from build123d import *

# Parameters (mm, degrees)
SKETCH1_R           = 7.95
BOSS_EXTRUDE1_DEPTH = 19.5
BOSS_EXTRUDE2_DEPTH = 1.5
SKETCH3_R           = 8.5
BOSS_EXTRUDE3_DEPTH = 2
BOSS_EXTRUDE3_TAPER = 30
SKETCH4_R           = 6
CUT_EXTRUDE1_DEPTH  = 2
SKETCH6_R           = 6
BOSS_EXTRUDE4_DEPTH = 2
BOSS_EXTRUDE4_TAPER = 30
SKETCH7_R           = 6.25
BOSS_EXTRUDE5_DEPTH = 9.3
SKETCH8_W           = 2.45599171
SKETCH8_H           = 0.676111723
SKETCH8_W_2         = 0.61301599
SKETCH8_H_2         = 2.333871056
SKETCH8_H_3         = 0.814342288
SKETCH8_W_3         = 0.602821575
BOSS_EXTRUDE6_DEPTH = 6


with BuildPart() as part:
    # Sketch1 → Boss-Extrude1 (new body)
    with BuildSketch(Plane(origin=(0, 0, 0), x_dir=(1, 0, 0), z_dir=(0, 1, 0))):
        with Locations(Location((0, 0, 0), (0, 0, 270))):
            Circle(SKETCH1_R)
    extrude(amount=BOSS_EXTRUDE1_DEPTH)

    # Sketch2 → Boss-Extrude2 (add)
    with BuildSketch(Plane(origin=(0, 19.5, 0), x_dir=(1, 0, 0), z_dir=(0, 1, 0))):
        Polygon((11.547005384, 0), (5.773502692, 10), (-5.773502692, 10), (-11.547005384, 0), (-5.773502692, -10), (5.773502692, -10), align=None)
    extrude(amount=-BOSS_EXTRUDE2_DEPTH)

    # Sketch3 → Boss-Extrude3 (add)
    with BuildSketch(Plane(origin=(0, 19.5, 0), x_dir=(1, 0, 0), z_dir=(0, 1, 0))):
        Circle(SKETCH3_R)
    extrude(amount=BOSS_EXTRUDE3_DEPTH, taper=BOSS_EXTRUDE3_TAPER)

    # Sketch4 → Cut-Extrude1 (cut)
    with BuildSketch(Plane(origin=(0, 21.5, 0), x_dir=(1, 0, 0), z_dir=(0, 1, 0))):
        with Locations(Location((0, 0, 0), (0, 0, 270))):
            Circle(SKETCH4_R)
    extrude(amount=-CUT_EXTRUDE1_DEPTH, mode=Mode.SUBTRACT)

    # Sketch6 → Boss-Extrude4 (add)
    with BuildSketch(Plane(origin=(0, 19.5, 0), x_dir=(1, 0, 0), z_dir=(0, 1, 0))):
        with Locations(Location((0, 0, 0), (0, 0, 270))):
            Circle(SKETCH6_R)
    extrude(amount=BOSS_EXTRUDE4_DEPTH, taper=BOSS_EXTRUDE4_TAPER)

    # Sketch7 → Boss-Extrude5 (add)
    with BuildSketch(Plane.XZ):
        with Locations(Location((0, 0, 0), (0, 0, 90))):
            Circle(SKETCH7_R)
    extrude(amount=BOSS_EXTRUDE5_DEPTH)

    # Sketch8 → Boss-Extrude6 (add)
    with BuildSketch(Plane.XZ.offset(9.3)):
        with Locations((0, 4.683948284)):
            Rectangle(SKETCH8_W, SKETCH8_H)
        with Locations((5.389572467, 0)):
            Rectangle(SKETCH8_W_2, SKETCH8_H_2)
        with Locations((0, -4.982726266)):
            Rectangle(SKETCH8_W, SKETCH8_H_3)
        with Locations((-4.707688923, 0)):
            Rectangle(SKETCH8_W_3, SKETCH8_H_2)
    extrude(amount=BOSS_EXTRUDE6_DEPTH)


solid = part.part
Source: CAD feature listing. Evaluate the final solid. Frame: model axes, mm. A direction names the side the tool comes from. Coordinates: 2 decimals unless noted, no trailing zeros. Loops run counter-clockwise (first coordinate to the right, second up) from the corner with the lowest first, then second, coordinate; pieces in that order, holes last. Notation, with made-up numbers: M 25,36 L 33,36 A21 ccw 33,74 Z; hole C 58,56 d5. An arc over 180 degrees is marked long. Answer in a Markdown table with one row per item.
Q1. Ray query, probe 1 along Y at (x, z) = (8, -5); probe 2 along Y at (x, z) = (4.75, -5.5); probe 3 along X at (y, z) = (17.5, -0.25). Return the intervals inside material, ascending. Write a range as from..to.
Answers below:
| item | result |
|---|---|
| probe 1 | y = 18..19.5 |
| probe 2 | y = 0..21.5 |
| probe 3 | x = -7.95..7.95 |
Q2. Section B-B on x = 10. Return the cut outline in (y, z).
Answers below:
| item | result |
|---|---|
| outline | M 18,-2.68 L 19.5,-2.68 L 19.5,2.68 L 18,2.68 Z |
Q3. Draft query along Z for faces 4 (the flat face through (0, -12, -4.576)), 5 (the flat face through (-5.009, -12, 0)), 6 (the flat face through (0, 19, -10)). Return one class per face: pulls with the +Z half, pulls with the -Z half, needs draft (parallel to the pull), parting line crosses it, or undercut.
Answers below:
| item | result |
|---|---|
| face 4 | undercut |
| face 5 | needs draft |
| face 6 | pulls with the -Z half |
Q4. First-contact query: pin 1 (0.7 mm diameter, centred on x = 0, y = -11.5, fed in from -Z); pin 2 (1.9 mm diameter, centred on y = -12.5, z = 0, fed in from +X); pin 3 (6 mm diameter, centred on y = 2, z = 5, fed in from +X); pin 4 (11 mm diameter, centred on x = 0, z = 0, fed in from -Y). Flat tips, straight axial feed; report the tip coordinate or a pass-through.
Answers below:
| item | result |
|---|---|
| pin 1 | stops at z = -5.39 |
| pin 2 | stops at x = 5.7 |
| pin 3 | stops at x = 7.69 |
| pin 4 | stops at y = -15.3 |
Q5. Set-up query: faces 1 (the flat face through (5.696, -12, 0)), 2 (the flat face through (6.8, 18, -4.5)), 3 (the flat face through (-1.228, -12, -5)). Return all of +Z, -Z, +X, -X, +Y, -Y with unobstructed straight access to the full face (end or side cutting, diameter ignored); none if empty.
Answers below:
| item | result |
|---|---|
| face 1 | +Z, -Z, +X, -Y |
| face 2 | -Y |
| face 3 | +Z, -Z, -X, -Y |
Q6. Section A-A on y = 15. Return the cut outline in (x, z), plus the area to 3 significant figures.
Answers below:
| item | result |
|---|---|
| outline | C 0,0 d15.9 |
| area | 199 mm^2 |
